from build123d import *

# Parameters (mm, degrees)
F0_W     = 10
F0_H     = 100
F1_DEPTH = 1800
F4_D     = 6


with BuildPart() as f1:
    # F0 (on Front) → F1 (new body)
    with BuildSketch(Plane.XZ):
        with Locations((14.071317, 54.374899)):
            Rectangle(F0_W, F0_H)
    extrude(amount=-F1_DEPTH)

    # F4 (through all)
    with Locations(Plane.YZ.offset(19.071317)):
        with Locations((20, 79.374899), (20, 19.374899), (74.147792, 84.374899), (83.515501, 24.374899)):
            Hole(F4_D / 2)


solid = f1.part
Work out the finished part from the listing and answer in its coordinate system (mm). Coordinates: 2 decimals unless noted, no trailing zeros.
1. For a pull along X with two mould halves and no side action, classify faces 1 (the flat face through (9.071, 887, 54)), 2 (the flat face through (19.071, 887, 54)) as +X half, -X half, draft (parallel to the pull), parting line (faces both ways), or undercut.
Results list:
face 1: -X half
face 2: +X half
2. A flat-ended cylindrical pin translates along its axis: pin 1 (5 mm diameter, centred on y = 83.52, z = 24.37, fed in from -X). Find the tip coordinate at first contact, or state that the pin passes through.
Results list:
pin 1: passes through
3. Consider line 1 along Z through (x, y) = (15.25, 20); line 2 along Y through (x, z) = (12.5, 82); line 3 along Y through (x, z) = (14, 25.5). Determine where each line is inside the solid, lowest interval first.
Results list:
line 1: z = 4.37 to 16.37, 22.37 to 76.37, 82.37 to 104.37
line 2: y = 0 to 18.55, 21.45 to 72.31, 75.98 to 1800
line 3: y = 0 to 80.73, 86.3 to 1800
